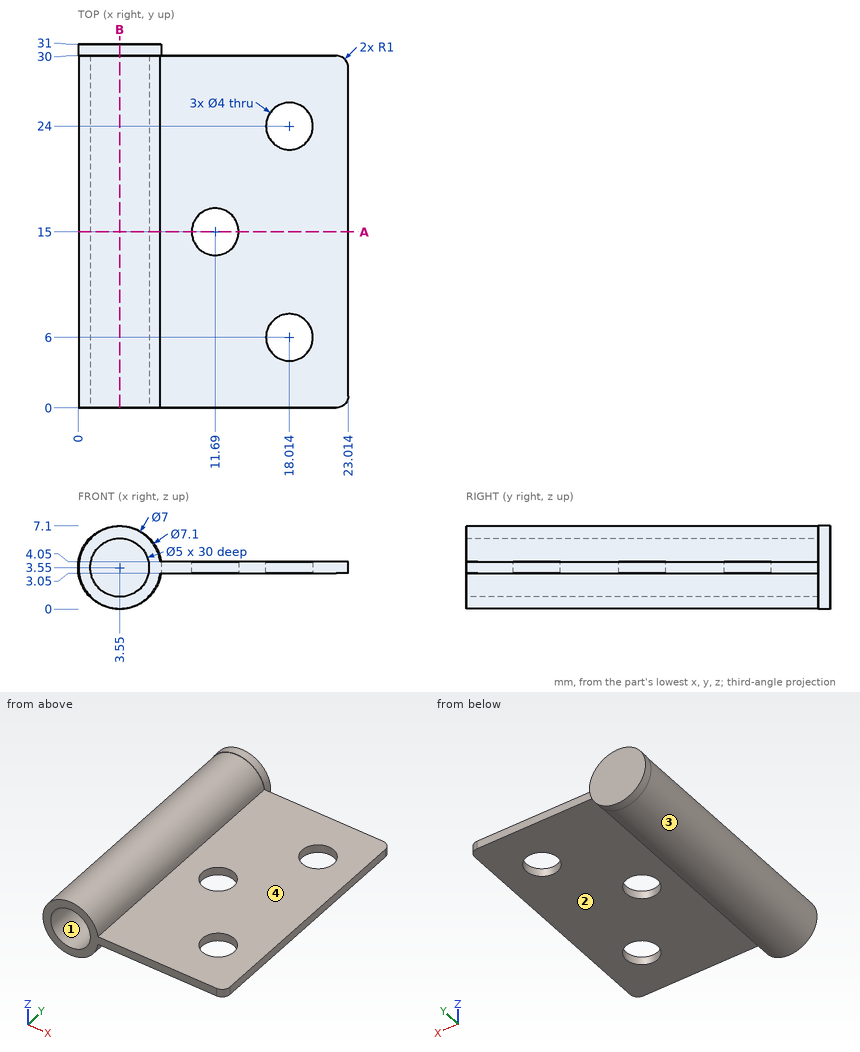
For this review, use the dimensioned drawing (mm, ordinates from the lowest corner) and the shaded views. Give positions to 0.01 mm unless a question says otherwise; leave off trailing zeros. Write each loop counter-clockwise with the first axis right and the second up, starting at its lowest first coordinate (ties: lowest second). Pieces come first, ordered by that corner, then holes. Notation, with made-up numbers: M 64,39.25 L 80,39.25 A13 ccw 80,43.25 Z; hole C 12,19.25 d2. An arc over 180 degrees is marked long. Answer as a JSON object with one key per item and string values. Group by question number.
Item 1: For probe 1 along Z at (x, y) = (3.5, 18.5); probe 2 along Y at (x, z) = (2.5, 1.5); probe 3 along X at (y, z) = (3, 3.75) (1 decimal), list the stretches that pass through material, from the lowest coordinate up. Write a range as [from, to].
Item 2: For pin 1 Ø5 at (x, y) = (19, 24) entering from +Z; pin 2 Ø1.1 at (x, z) = (17, 3.5) entering from +Y; pin 3 Ø6.5 at (x, y) = (18.01, 6) entering from -Z, all flat-tipped, find the tip position at first contact; note any pin that passes through.
Item 3: Draft analysis for pull direction Z (two halves, no side actions). For the marked faces 1, 2, 3 and 4, state which applies: +Z half, -Z half, draft (parallel to the pull), parting line (faces both ways), or undercut.
Item 4: Consider section B-B on x = 3.55. Write out the cut boundary in (y, z).
Item 5: Consider section A-A on y = 15. Count the separate pieces of the cut face and the enclosed holes in it.
Check result:
{
 "1": {"probe 1": "z = [0.05, 1.05], [6.05, 7.05]", "probe 2": "y = [30, 31]", "probe 3": "x = [0.1, 1.1], [6, 23]"},
 "2": {"pin 1": "stops at z = 4.05", "pin 2": "stops at y = 30", "pin 3": "stops at z = 3.05"},
 "3": {"face 1": "undercut", "face 2": "-Z half", "face 3": "parting line", "face 4": "+Z half"},
 "4": {"outline": "M 0,0.05 L 30,0.05 L 30,0 L 31,0 L 31,7.1 L 30,7.1 L 30,7.05 L 0,7.05 L 0,6.05 L 30,6.05 L 30,1.05 L 0,1.05 Z"},
 "5": {"separate pieces": "2", "enclosed holes": "1"}
}
